from build123d import *

# Parameters (mm, degrees)
SKETCH3_R           = 10.16
CUT_EXTRUDE1_DEPTH  = 2.54
SKETCH5_R           = 4.7625
CUT_EXTRUDE2_DEPTH  = 6.35
SKETCH11_R          = 0.889
CUT_EXTRUDE6_DEPTH  = 55.372
SKETCH12_R          = 28.194
SKETCH12_R_2        = 26.924
BOSS_EXTRUDE1_DEPTH = 2.54


with BuildPart() as part:
    # Sketch2 → Revolve1 (revolve)
    with BuildSketch(Plane(origin=(0, 0, 0), x_dir=(0, 0, -1), z_dir=(1, 0, 0))):
        Polygon((-6.35, 42.32529), (0, 42.32529), (0, 47.625), (2.54, 47.625), (2.54, 0), (0, 0), (0, 39.839805153), (-8.89, 39.839805153), (-8.89, 47.625), (-6.35, 47.625), align=None)
    revolve(axis=Axis((0, 0, 0), (0, 0, -1)))

    # Sketch3 → Cut-Extrude1 (cut)
    with BuildSketch(Plane.XY):
        Circle(SKETCH3_R)
    extrude(amount=-CUT_EXTRUDE1_DEPTH, mode=Mode.SUBTRACT)

    # Sketch5 → Cut-Extrude2 (cut)
    with BuildSketch(Plane.XY):
        with Locations((0, 22.225)):
            Circle(SKETCH5_R)
    extrude(amount=-CUT_EXTRUDE2_DEPTH, mode=Mode.SUBTRACT)

    # Sketch11 → Cut-Extrude6 (cut)
    with BuildSketch(Plane(origin=(0, 0, 0), x_dir=(1, 0, 0), z_dir=(0, 1, 0))):
        with Locations((0, -3.870418615)):
            Circle(SKETCH11_R)
    extrude(amount=CUT_EXTRUDE6_DEPTH, mode=Mode.SUBTRACT)

    # Sketch12 → Boss-Extrude1 (add)
    with BuildSketch(Plane(origin=(0, 0, -2.54), x_dir=(-1, 0, 0), z_dir=(0, 0, -1))):
        Circle(SKETCH12_R)
        Circle(SKETCH12_R_2, mode=Mode.SUBTRACT)
    extrude(amount=BOSS_EXTRUDE1_DEPTH)


solid = part.part
Verification items for the finished model (mm, model axes). A direction names the side the tool comes from. Coordinates: 2 decimals unless noted, no trailing zeros. Order: outer loops, then holes, each group sorted by start corner. A loop starts at its lowest first (then second) coordinate and runs counter-clockwise, first axis right, second up.
1. Sectioned sample at C-C, the plane y = 15. Record the cut outline in (x, z), and give its area (3 significant figures).
Results found:
outline: (-45.2, -2.54) - (-23.87, -2.54) - (-23.87, -5.08) - (-22.36, -5.08) - (-22.36, -2.54) - (22.36, -2.54) - (22.36, -5.08) - (23.87, -5.08) - (23.87, -2.54) - (45.2, -2.54) - (45.2, 0) - (39.58, 0) - (39.58, 6.35) - (45.2, 6.35) - (45.2, 8.89) - (36.91, 8.89) - (36.91, 0) - (-36.91, 0) - (-36.91, 8.89) - (-45.2, 8.89) - (-45.2, 6.35) - (-39.58, 6.35) - (-39.58, 0) - (-45.2, 0) - close
area: 313 mm2
2. Set-up check for faces 1 (the face through (21.37, -16.38, -3.79)), 2 (the face through (12.71, 40.37, 3.13)), 3 (the face through (-24.242, -31.616, 4.507)): record each of +Z, -Z, +X, -X, +Y, -Y from which the full face is reachable in a straight line by a thin tool's end or side.
Results found:
face 1: -Z
face 2: none
face 3: +Z
3. Release check for a two-part mould opening along X. For faces 4 (the face through (-1.323, 10.074, -1.252)), 5 (the face through (43, 0, 6.35)), 6 (the face through (-28.979, -37.794, -1.288)) record: +X half, -X half, draft (parallel to the pull), parting line (faces both ways), or undercut.
Results found:
face 4: undercut
face 5: draft
face 6: parting line
4. Sectioned sample at B-B, the plane x = 36. Record the cut outline in (y, z).
Results found:
outline: (-31.18, -2.54) - (31.18, -2.54) - (31.18, 0) - (22.26, 0) - (22.26, 6.35) - (31.18, 6.35) - (31.18, 8.89) - (17.06, 8.89) - (17.06, 0) - (-17.06, 0) - (-17.06, 8.89) - (-31.18, 8.89) - (-31.18, 6.35) - (-22.26, 6.35) - (-22.26, 0) - (-31.18, 0) - close
5. Go/stop test with flat-tipped pins: pin 1 Ø5 at (y, z) = (12, 1) entering from -X; pin 2 Ø1.5 at (x, z) = (18, -0.5) entering from -Y; pin 3 Ø1 at (x, z) = (-5, 3.5) entering from -Y; pin 4 Ø8.5 at (x, y) = (0, 22.225) entering from -Z. Record where each tip stops, or that it passes through.
Results found:
pin 1: stops at x = -46.62
pin 2: stops at y = -44.39
pin 3: stops at y = -42.09
pin 4: passes through
6. Sectioned sample at D-D, the plane y = -17. Record the cut outline in (x, z), and give its area (3 significant figures).
Results found:
outline: (-44.49, -2.54) - (-22.49, -2.54) - (-22.49, -5.08) - (-20.88, -5.08) - (-20.88, -2.54) - (20.88, -2.54) - (20.88, -5.08) - (22.49, -5.08) - (22.49, -2.54) - (44.49, -2.54) - (44.49, 0) - (38.76, 0) - (38.76, 6.35) - (44.49, 6.35) - (44.49, 8.89) - (36.03, 8.89) - (36.03, 0) - (-36.03, 0) - (-36.03, 8.89) - (-44.49, 8.89) - (-44.49, 6.35) - (-38.76, 6.35) - (-38.76, 0) - (-44.49, 0) - close
area: 312 mm2
7. Scan lines: line 1 (X direction, y = 0, z = 3); line 2 (Z direction, x = -28, y = 35.5); line 3 (Y direction, x = 0, z = -3.15). Record each from-to range of solid material in increasing order.
Results found:
line 1: x = -42.33 to -39.84, 39.84 to 42.33
line 2: z = -2.54 to 0, 6.35 to 8.89
line 3: y = -28.19 to -26.92, 26.92 to 28.19
8. Sectioned sample at A-A, the plane y = 0. Record the cut outline in (x, z) (3 decimals), and give its area (3 significant figures).
Results found:
outline: (-47.625, -2.54) - (-28.194, -2.54) - (-28.194, -5.08) - (-26.924, -5.08) - (-26.924, -2.54) - (-10.16, -2.54) - (-10.16, 0) - (-39.84, 0) - (-39.84, 8.89) - (-47.625, 8.89) - (-47.625, 6.35) - (-42.325, 6.35) - (-42.325, 0) - (-47.625, 0) - close; (10.16, -2.54) - (26.924, -2.54) - (26.924, -5.08) - (28.194, -5.08) - (28.194, -2.54) - (47.625, -2.54) - (47.625, 0) - (42.325, 0) - (42.325, 6.35) - (47.625, 6.35) - (47.625, 8.89) - (39.84, 8.89) - (39.84, 0) - (10.16, 0) - close
area: 268 mm2
